Work out the finished part from the listing and answer in its coordinate system (mm). Face numbers are marked on the shaded views. A direction names the side the tool comes from. Round coordinates to 2 decimals unless told otherwise and drop trailing zeros. Write each loop counter-clockwise with the first axis right and the second up, starting at its lowest first coordinate (ties: lowest second). Pieces come first, ordered by that corner, then holes.
from build123d import *

# Parameters (mm, degrees)
F1_DEPTH = 52
F3_DEPTH = 20
F5_DEPTH = 25
F6_R     = 26
F7_R     = 25.99999


# Not quite as in the source:
# - a fillet or chamfer is up to 0.001 mm smaller than in the source, because OpenCascade refuses the exact size


with BuildPart() as f1:
    # F0 (on Front) → F1 (new body)
    with BuildSketch(Plane.XZ):
        Polygon((-38.2547932683, -20), (-38.2547932683, 0), (-35.5326342583, 0), (-29.9705220208, 0), (-94.8233357632, 64.8528137424), (-108.9654713869, 50.7106781187), align=None)
        Polygon((-35.5326342583, 0), (-38.2547932683, 0), (-38.2547932683, -20), (-9.9705220208, -20), (-29.9705220208, 0), align=None)
        Polygon((81.7452067317, 0), (-29.9705220208, 0), (-9.9705220208, -20), (81.7452067317, -20), align=None)
    extrude(amount=F1_DEPTH)

    # F2 (on face) → F3 (cut)
    with BuildSketch(Plane.XY):
        with BuildLine():
            Line((-18.2547932683, -36), (61.7452067317, -36))
            ThreePointArc((61.7452067317, -36), (68.8162745436, -33.0710678119), (71.7452067317, -26))
            ThreePointArc((71.7452067317, -26), (68.8162745436, -18.9289321881), (61.7452067317, -16))
            Line((61.7452067317, -16), (-18.2547932683, -16))
            ThreePointArc((-18.2547932683, -16), (-28.2547932683, -26), (-18.2547932683, -36))
        make_face()
    extrude(amount=-F3_DEPTH, mode=Mode.SUBTRACT)

    # F4 (on face) → F5 (cut)
    with BuildSketch(Plane(origin=(-14.9852610104, 0, -14.9852610104), x_dir=(0, 1, 0), z_dir=(0.7071067812, 0, 0.7071067812))):
        with BuildLine():
            ThreePointArc((-16.4961378883, 86.9204033326), (-19.2517821929, 93.8138285014), (-26, 96.9080881091))
            Line((-26, 96.9080881091), (-26.9922757766, 96.9080881091))
            ThreePointArc((-26.9922757766, 96.9080881091), (-33.3895630572, 79.6760476372), (-16.4961378883, 86.9204033326))
        make_face()
    extrude(amount=-F5_DEPTH, mode=Mode.SUBTRACT)

    # F6
    f6_edges = [f1.edges().sort_by_distance(p)[0] for p in [
        (-101.894404, -52, 57.781746),
    ]]
    fillet(f6_edges, radius=F6_R)

    # F7 (radius 26 in the source; OpenCascade refuses exactly that, so slightly less here)
    f7_edges = [f1.edges().sort_by_distance(p)[0] for p in [
        (-101.894404, 0, 57.781746),
    ]]
    fillet(f7_edges, radius=F7_R)


solid = f1.part
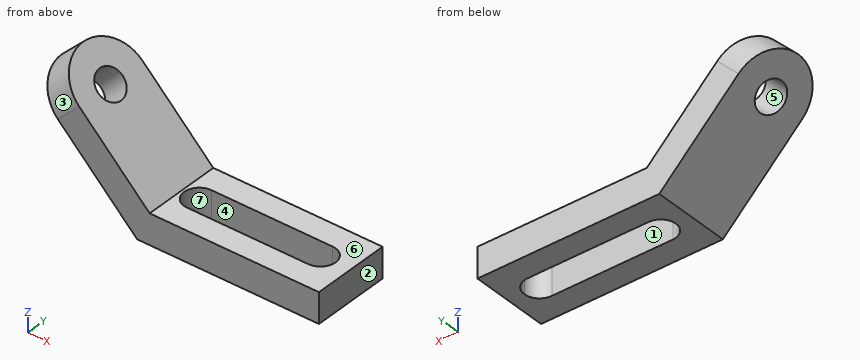
Q1. Find section C-C (y = -13.5). Determine the outline of the cut face in (x, z), plus the area to 3 significant figures.
Q2. Find section A-A (y = -31). Determine the outline of the cut face in (x, z), plus the area to 3 significant figures.
Q3. Given pin 1 (1 mm diameter, centred on y = -45, z = 24.5, fed in from +X); pin 2 (1.5 mm diameter, centred on x = 26.5, y = -44, fed in from +Z); pin 3 (6 mm diameter, centred on y = -33.5, z = -5, fed in from -X), each flat-ended and moving along its own axis, determine where each tip first touches the part or whether it passes through.
Q4. Find section B-B (z = -6). Determine the outline of the cut face in (x, y), plus the area to 3 significant figures.
Q5. Find section D-D (z = 9.5). Determine the outline of the cut face in (x, y), plus the area to 3 significant figures.
Q6. The mould has two halves that part along X. Classify the marked faces 1, 2, 3 and 4: +X half, -X half, draft (parallel to the pull), parting line (faces both ways), or undercut.
Q7. A tool of negligible diameter and unlimited length cuts with its end or side. For the marked faces 5, 6 and 7, from which of +Z, -Z, +X, -X, +Y, -Y can it reach the whole face along a straight path? Write none if from no direction.
Q8. Find the intervals of material crossed by L1, parallel to Y at x = -1.5, z = -11; L2, parallel to Z at x = 37.5, y = -10; L3, parallel to Z at x = -90, y = -13, in increasing order.
Report:
1. outline: (-106.7, 48.45) - (-38.25, -20) - (81.75, -20) - (81.75, 0) - (-29.97, 0) - (-92.56, 62.59) - close
1. area: 4,170 mm2
2. outline: (-108.62, 50.37) - (-96.9, 38.65) - (-82.76, 52.79) - (-94.48, 64.51) - close; (-84.28, 26.02) - (-38.25, -20) - (-26.92, -20) - (-26.92, 0) - (-29.97, 0) - (-70.13, 40.16) - close; (70.41, -20) - (81.75, -20) - (81.75, 0) - (70.41, 0) - close
2. area: 1,920 mm2
3. pin 1: stops at x = -53.97
3. pin 2: stops at z = 0
3. pin 3: stops at x = -56.25
4. outline: (-52.25, -52) - (81.75, -52) - (81.75, 0) - (-52.25, 0) - close; hole (-18.25, -36) - (61.75, -36) arc R10 ccw to (61.75, -16) - (-18.25, -16) arc R10 ccw to start
4. area: 5,050 mm2
5. outline: (-67.75, -52) - (-39.47, -52) - (-39.47, 0) - (-67.75, 0) - close
5. area: 1,470 mm2
6. face 1: undercut
6. face 2: +X half
6. face 3: -X half
6. face 4: undercut
7. face 5: none
7. face 6: +Z, +X, +Y, -Y
7. face 7: +Z, -Z
8. L1: y = -52 to -36, -16 to 0
8. L2: z = -20 to 0
8. L3: z = 31.75 to 60.03
